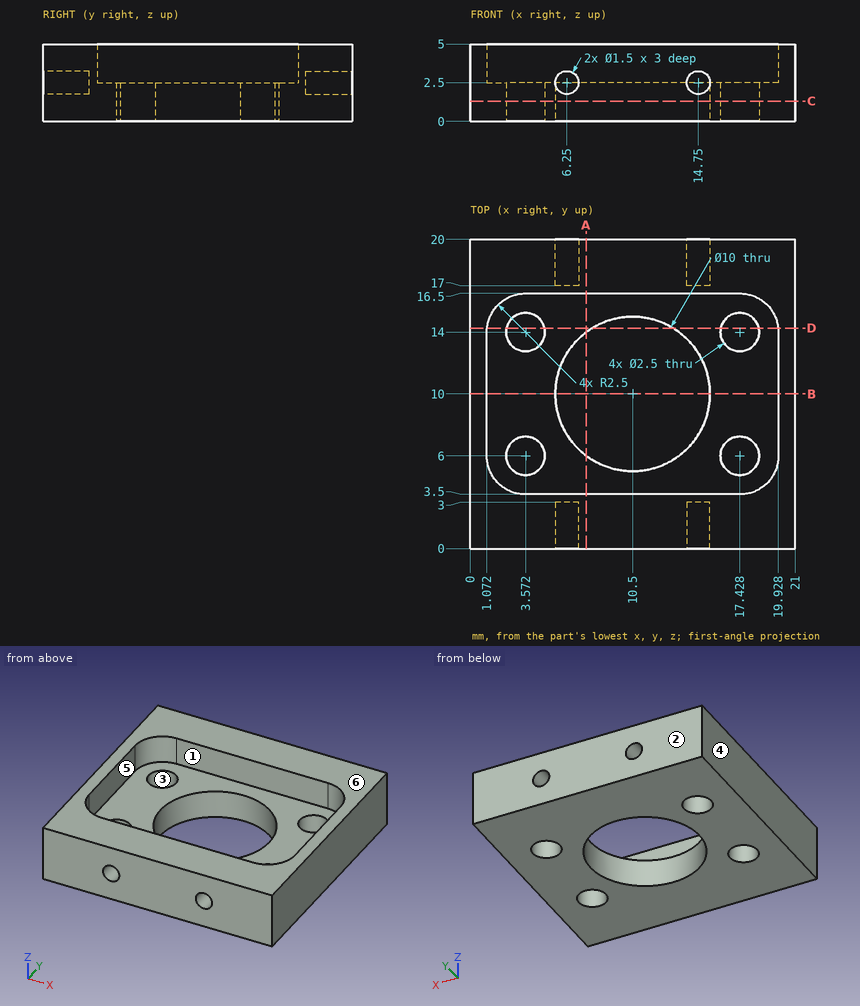
Job drawing, mm, ordinate dimensions from the low corner. One solid piece. A direction names the side the tool comes from. Coordinates: 2 decimals unless noted, no trailing zeros. Write each loop counter-clockwise with the first axis right and the second up, starting at its lowest first coordinate (ties: lowest second). Pieces come first, ordered by that corner, then holes.
Item 1: Pin check, flat tips, straight feed: pin 1 (4 mm diameter, centred on x = 3.57, y = 14, fed in from +Z); pin 2 (0.8 mm diameter, centred on x = 14.5, z = 2.5, fed in from +Y); pin 3 (1.4 mm diameter, centred on x = 14.75, z = 2.5, fed in from -Y). Stop position of each tip, or through.
Item 2: Probe line 1 (X direction, y = 18.85, z = 2.5); line 2 (Y direction, x = 17.5, z = 1.9); line 3 (X direction, y = 14, z = 2.6). List the from-to ranges inside material, lowest first.
Item 3: Slice it at B-B (y = 10). Write the cut outline in (x, z).
Item 4: Slice it at C-C (z = 1.3). Write the cut outline in (x, y).
Item 5: Slice it at D-D (y = 14.25). Write the cut outline in (x, z), and give its area (3 significant figures).
Item 6: Which spindle directions (+Z, -Z, +X, -X, +Y, -Y) get a long thin tool onto all of the face, cutting with end or side? Do the marked faces 1 and 2. Say none if no direction does.
Item 7: Slice it at A-A (x = 7.5). Write the cut outline in (y, z).
Item 8: Mould opens along X. For the marked faces 3, 4, 5 and 6 say: released by +X, released by -X, zero draft, split by the parting line, or undercut.
Results found:
1. pin 1: stops at z = 2.5
1. pin 2: stops at y = 17
1. pin 3: stops at y = 3
2. line 1: x = 0 to 5.5, 7 to 14, 15.5 to 21
2. line 2: y = 0 to 4.75, 7.25 to 12.75, 15.25 to 20
2. line 3: x = 0 to 1.07, 19.93 to 21
3. outline: (0, 0) - (5.5, 0) - (5.5, 2.5) - (1.07, 2.5) - (1.07, 5) - (0, 5) - close; (15.5, 0) - (21, 0) - (21, 5) - (19.93, 5) - (19.93, 2.5) - (15.5, 2.5) - close
4. outline: (0, 0) - (21, 0) - (21, 20) - (0, 20) - close; hole circle Ø2.5 at (3.57, 6); hole circle Ø2.5 at (3.57, 14); hole circle Ø10 at (10.5, 10); hole circle Ø2.5 at (17.43, 6); hole circle Ø2.5 at (17.43, 14)
5. outline: (0, 0) - (2.35, 0) - (2.35, 2.5) - (1.08, 2.5) - (1.08, 5) - (0, 5) - close; (4.8, 0) - (7.87, 0) - (7.87, 2.5) - (4.8, 2.5) - close; (13.13, 0) - (16.2, 0) - (16.2, 2.5) - (13.13, 2.5) - close; (18.65, 0) - (21, 0) - (21, 5) - (19.92, 5) - (19.92, 2.5) - (18.65, 2.5) - close
5. area: 32.5 mm2
6. face 1: +Z
6. face 2: +Z, -Z, +X, -X, +Y
7. outline: (0, 0) - (6, 0) - (6, 2.5) - (3.5, 2.5) - (3.5, 5) - (0, 5) - close; (14, 0) - (20, 0) - (20, 5) - (16.5, 5) - (16.5, 2.5) - (14, 2.5) - close
8. face 3: undercut
8. face 4: released by -X
8. face 5: undercut
8. face 6: zero draft
